Could you check a few things on this model? Use its own coordinates, in mm. Face numbers are marked on the shaded views. A direction names the side the tool comes from. Give positions to 0.01 mm unless a question says otherwise; leave off trailing zeros. Loops run counter-clockwise (first coordinate to the right, second up) from the corner with the lowest first, then second, coordinate; pieces in that order, holes last. Notation, with made-up numbers: M 50,32 L 75,32 A26 cw 75,60 Z; hole C -3,63.25 d9. An arc over 180 degrees is marked long. Answer in a Markdown table with one row per item. Add a question column.
Autodesk Inventor part; units mm, degrees
ref_plane "YZ Plane" through (0, 0, 0) normal (1, 0, 0) x (0, 1, 0)
ref_plane "XZ Plane" through (0, 0, 0) normal (0, 1, 0) x (-1, 0, 0)
ref_plane "XY Plane" through (0, 0, 0) normal (0, 0, 1) x (1, 0, 0)
sketch "Sketch1" plane through (0, 0, 0) normal (0, 0, 1) x (1, 0, 0)
  line L0 (-9.5263, 5.5) -> (-17.3205, 10)
  line L1 (0, 0) -> (20, 0) construction
  line L2 (-9.5263, -5.5) -> (-17.3205, -10)
  line L3 (0, 0) -> (20, 0) construction
  line L4 (5.5, 9.5263) -> (10, 17.3205)
  line L5 (0, 0) -> (20, 0) construction
  line L6 (-5.5, 9.5263) -> (-10, 17.3205)
  line L7 (0, 0) -> (20, 0) construction
  line L8 (5.5, -9.5263) -> (10, -17.3205)
  line L9 (-5.5, -9.5263) -> (-10, -17.3205)
  line L10 (0, 0) -> (0, 20) construction
  line L11 (9.5263, 5.5) -> (17.3205, 10)
  line L12 (9.5263, -5.5) -> (17.3205, -10)
  arc A0 (17.3205, 10) -> (10, 17.3205) centre (0, 0) ccw
  arc A1 (-10, 17.3205) -> (-17.3205, 10) centre (0, 0) ccw
  arc A2 (-17.3205, -10) -> (-10, -17.3205) centre (0, 0) ccw
  arc A3 (10, -17.3205) -> (17.3205, -10) centre (0, 0) ccw
  arc A4 (-9.5263, 5.5) -> (-9.5263, -5.5) centre (0, 0) ccw
  arc A5 (5.5, 9.5263) -> (-5.5, 9.5263) centre (0, 0) ccw
  arc A6 (-5.5, -9.5263) -> (5.5, -9.5263) centre (0, 0) ccw
  arc A7 (9.5263, -5.5) -> (9.5263, 5.5) centre (0, 0) ccw
  dimension "d2" = 150
  dimension "d3" = 150
  dimension "d4" = 60
  dimension "d5" = 120
extrude "Extrusion1" add sketch "Sketch1" along normal blind 10
properties part number "NYLON-JAW"
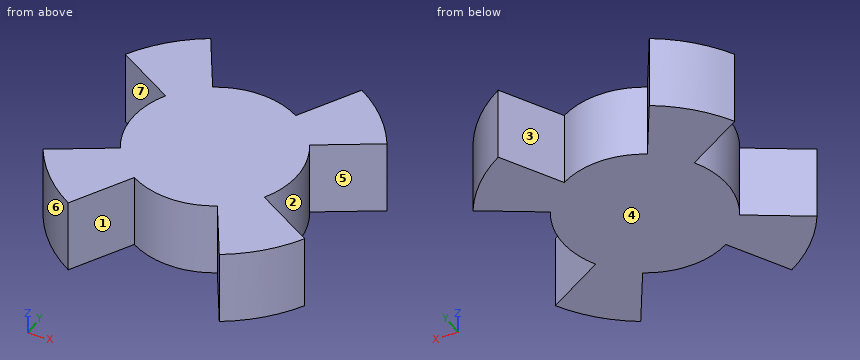
Item 1: Suppose I cut it at D-D (x = -15). List the corners of the cut face in (y, z) for me, then the cut area to 3 significant figures.
Item 2: For the marked faces 5, 6 and 7, which set-ups out of +Z, -Z, +X, -X, +Y, -Y let a thin tool reach every point of the face, with its end or its side?
Item 3: I need wall thicknesses on L1, parallel to X at y = -12, z = 1.25; L2, parallel to X at y = 15, z = 3; L3, parallel to Y at x = 1.5, z = 4. Which ranges of each line are inside material? Lowest first, please.
Item 4: For P1, Ø5, axis at x = -6.5, z = 7, coming from the +Y side; P2, Ø5, axis at x = -4, z = 2.5, coming from the -Y side; P3, Ø1.5, axis at y = -6.5, z = 4.5, coming from the -X side, each with a flat end and sliding along its axis, tell me the tip position at first contact or that it passes through.
Item 5: If we mould it in two halves opening along Y, with no side actions, what happens to the marked faces 1, 2, 3 and 4? For each: +Y half, -Y half, draft (parallel to the pull), parting line (faces both ways), or undercut.
Item 6: Suppose I cut it at B-B (z = 6.75). List the corners of the cut face in (x, y) for me.
Item 7: Suppose I cut it at C-C (y = 14). List the corners of the cut face in (x, z) for me, then the cut area to 3 significant figures.
Item 8: Suppose I cut it at A-A (x = 10.5). List the corners of the cut face in (y, z) for me.
Values found:
| question | item | result |
|---|---|---|
| 1 | outline | M -13.23,0 L -8.66,0 L -8.66,10 L -13.23,10 Z; M 8.66,0 L 13.23,0 L 13.23,10 L 8.66,10 Z |
| 1 | area | 91.4 mm² |
| 2 | face 5 | +Z, -Z, +X |
| 2 | face 6 | +Z, -Z, -X, -Y |
| 2 | face 7 | +Z, -Z, -X |
| 3 | L1 | -16 to -6.93, 6.93 to 16 |
| 3 | L2 | -13.23 to -8.66, 8.66 to 13.23 |
| 3 | L3 | -10.9 to 10.9 |
| 4 | P1 | y = 15.59 |
| 4 | P2 | y = -11.26 |
| 4 | P3 | x = -12.56 |
| 5 | face 1 | -Y half |
| 5 | face 2 | undercut |
| 5 | face 3 | +Y half |
| 5 | face 4 | draft |
| 6 | outline | M -17.32,-10 A20 ccw -10,-17.32 L -5.5,-9.53 A11 ccw 5.5,-9.53 L 10,-17.32 A20 ccw 17.32,-10 L 9.53,-5.5 A11 ccw 9.53,5.5 L 17.32,10 A20 ccw 10,17.32 L 5.5,9.53 A11 ccw -5.5,9.53 L -10,17.32 A20 ccw -17.32,10 L -9.53,5.5 A11 ccw -9.53,-5.5 Z |
| 7 | outline | M -14.28,0 L -8.08,0 L -8.08,10 L -14.28,10 Z; M 8.08,0 L 14.28,0 L 14.28,10 L 8.08,10 Z |
| 7 | area | 124 mm² |
| 8 | outline | M -17.02,0 L -6.06,0 L -6.06,10 L -17.02,10 Z; M -3.28,0 L 3.28,0 L 3.28,10 L -3.28,10 Z; M 6.06,0 L 17.02,0 L 17.02,10 L 6.06,10 Z |
